from build123d import *

# Parameters (mm, degrees)
SKETCH1_W           = 736.6
SKETCH1_H           = 184.15
BOSS_EXTRUDE1_DEPTH = 38.1
CUT_EXTRUDE2_DEPTH  = 761.225224851
CHAMFER1_SIZE       = 2.54
CHAMFER2_SIZE       = 2.54
SKETCH2_R           = 19.05
CUT_EXTRUDE1_DEPTH  = 3.175


with BuildPart() as part:
    # Sketch1 → Boss-Extrude1 (new body)
    with BuildSketch(Plane(origin=(0, 0, 0), x_dir=(1, 0, 0), z_dir=(0, 1, 0))):
        with Locations((368.3, 92.075)):
            Rectangle(SKETCH1_W, SKETCH1_H)
        with BuildLine():
            Line((409.5623, 110.83925), (457.1238, 110.83925))
            ThreePointArc((457.1238, 110.83925), (469.8238, 98.13925), (457.1238, 85.43925))
            Line((457.1238, 85.43925), (409.5623, 85.43925))
            ThreePointArc((409.5623, 85.43925), (396.8623, 98.13925), (409.5623, 110.83925))
        make_face(mode=Mode.SUBTRACT)
    extrude(amount=BOSS_EXTRUDE1_DEPTH)

    # Sketch4 → Cut-Extrude2 (cut, through all)
    with BuildSketch(Plane.XZ):
        with BuildLine():
            Line((0, -184.15), (0, -113.957302712))
            ThreePointArc((0, -113.957302712), (2.738891811, -149.223945145), (8.343201677, -184.15))
            Line((8.343201677, -184.15), (0, -184.15))
        make_face()
    extrude(amount=-CUT_EXTRUDE2_DEPTH, mode=Mode.SUBTRACT)

    # Chamfer1
    # the kernel refuses this chamfer: 2.54 mm, written as the material it takes off along each edge
    with BuildSketch(Plane(origin=(736.6, 38.1, 6.532074789), x_dir=(0.027495876610568244, -0.9996219169112971, 0), z_dir=(0, 0, -1))) as chamfer1_piece_1:
        Polygon((CHAMFER1_SIZE * 0.999621916911, CHAMFER1_SIZE * 0.0274958766106), (-CHAMFER1_SIZE * 0.0274958766106, CHAMFER1_SIZE * 0.999621916911), (0, 0), align=None)
    extrude(amount=197.214149579, mode=Mode.SUBTRACT)
    with BuildSketch(Plane(origin=(457.1238, 38.1, -98.13925), x_dir=(0, 0, -1), z_dir=(-1, 0, 0))) as chamfer1_piece_2:
        Polygon((12.7 + CHAMFER1_SIZE, 0), (12.7, CHAMFER1_SIZE), (12.7, 0), align=None)
    revolve(axis=Axis((457.1238, 38.1, -98.13925), (0, -1, 0)), revolution_arc=180, mode=Mode.SUBTRACT)
    with BuildSketch(Plane(origin=(743.132074789, 38.1, -184.15), x_dir=(0, 0.027495876610587267, 0.9996219169112966), z_dir=(-1, 0, 0))) as chamfer1_piece_3:
        Polygon((CHAMFER1_SIZE * 0.999621916911, -CHAMFER1_SIZE * 0.0274958766106), (-CHAMFER1_SIZE * 0.0274958766106, -CHAMFER1_SIZE * 0.999621916911), (0, 0), align=None)
    extrude(amount=741.320947902, mode=Mode.SUBTRACT)
    with BuildSketch(Plane(origin=(409.5623, 38.1, -110.83925), x_dir=(0, 0.027495876610587267, -0.9996219169112966), z_dir=(1, 0, 0)), Plane(origin=(457.1238, 38.1, -85.43925), x_dir=(0, 0.027495876610587267, 0.9996219169112966), z_dir=(-1, 0, 0))) as chamfer1_piece_4:
        Polygon((CHAMFER1_SIZE * 0.999621916911, -CHAMFER1_SIZE * 0.0274958766106), (-CHAMFER1_SIZE * 0.0274958766106, -CHAMFER1_SIZE * 0.999621916911), (0, 0), align=None)
    extrude(amount=47.5615, mode=Mode.SUBTRACT)
    with BuildSketch(Plane(origin=(409.5623, 38.1, -98.13925), x_dir=(0, 0, 1), z_dir=(1, 0, 0))) as chamfer1_piece_5:
        Polygon((12.7 + CHAMFER1_SIZE, 0), (12.7, CHAMFER1_SIZE), (12.7, 0), align=None)
    revolve(axis=Axis((409.5623, 38.1, -98.13925), (0, -1, 0)), revolution_arc=180, mode=Mode.SUBTRACT)
    with BuildSketch(Plane(origin=(0, 38.1, -120.489377502), x_dir=(-0.02749587661058648, -0.9996219169112968, 0), z_dir=(0, 0, 1))) as chamfer1_piece_6:
        Polygon((CHAMFER1_SIZE * 0.999621916911, CHAMFER1_SIZE * 0.0274958766106), (-CHAMFER1_SIZE * 0.0274958766106, CHAMFER1_SIZE * 0.999621916911), (0, 0), align=None)
    extrude(amount=127.021452291, mode=Mode.SUBTRACT)
    with BuildSketch(Plane(origin=(433.324, 38.1, -98.044), x_dir=(-0.9997657983904642, 0, -0.021641357828885384), z_dir=(-0.021641357828885384, 0, 0.9997657983904642))) as chamfer1_piece_7:
        Polygon((433.6161 - CHAMFER1_SIZE, 0), (433.6161, CHAMFER1_SIZE), (433.6161, 0), align=None)
    revolve(axis=Axis((433.324, 38.1, -98.044), (0, -1, 0)), revolution_arc=11.076796252, mode=Mode.SUBTRACT)
    with BuildSketch(Plane(origin=(-6.532074789, 38.1, 0), x_dir=(0, -0.9996219169112968, 0.027495876610586393), z_dir=(1, 0, 0))) as chamfer1_piece_8:
        Polygon((CHAMFER1_SIZE * 0.999621916911, CHAMFER1_SIZE * 0.0274958766106), (-CHAMFER1_SIZE * 0.0274958766106, CHAMFER1_SIZE * 0.999621916911), (0, 0), align=None)
    extrude(amount=749.664149579, mode=Mode.SUBTRACT)

    # Chamfer2
    # the kernel refuses this chamfer: 2.54 mm, written as the material it takes off along each edge
    with BuildSketch(Plane(origin=(457.1238, 0, -98.13925), x_dir=(0, 0, -1), z_dir=(-1, 0, 0))) as chamfer2_piece_1:
        Polygon((12.7 + CHAMFER2_SIZE, 0), (12.7, -CHAMFER2_SIZE), (12.7, 0), align=None)
    revolve(axis=Axis((457.1238, 0, -98.13925), (0, -1, 0)), revolution_arc=180, mode=Mode.SUBTRACT)
    with BuildSketch(Plane(origin=(409.5623, 0, -110.83925), x_dir=(0, -0.027495876610586324, -0.9996219169112968), z_dir=(1, 0, 0)), Plane(origin=(457.1238, 0, -85.43925), x_dir=(0, -0.027495876610586324, 0.9996219169112968), z_dir=(-1, 0, 0))) as chamfer2_piece_2:
        Polygon((CHAMFER2_SIZE * 0.999621916911, CHAMFER2_SIZE * 0.0274958766106), (-CHAMFER2_SIZE * 0.0274958766106, CHAMFER2_SIZE * 0.999621916911), (0, 0), align=None)
    extrude(amount=47.5615, mode=Mode.SUBTRACT)
    with BuildSketch(Plane(origin=(409.5623, 0, -98.13925), x_dir=(0, 0, 1), z_dir=(1, 0, 0))) as chamfer2_piece_3:
        Polygon((12.7 + CHAMFER2_SIZE, 0), (12.7, -CHAMFER2_SIZE), (12.7, 0), align=None)
    revolve(axis=Axis((409.5623, 0, -98.13925), (0, -1, 0)), revolution_arc=180, mode=Mode.SUBTRACT)
    with BuildSketch(Plane(origin=(0, 0, -120.489377502), x_dir=(0.9996219169112968, -0.02749587661058605, 0), z_dir=(0, 0, 1))) as chamfer2_piece_4:
        Polygon((CHAMFER2_SIZE * 0.999621916911, CHAMFER2_SIZE * 0.0274958766106), (-CHAMFER2_SIZE * 0.0274958766106, CHAMFER2_SIZE * 0.999621916911), (0, 0), align=None)
    extrude(amount=127.021452291, mode=Mode.SUBTRACT)
    with BuildSketch(Plane(origin=(433.324, 0, -98.044), x_dir=(-0.9997657983904642, 0, -0.021641357828885415), z_dir=(-0.021641357828885415, 0, 0.9997657983904642))) as chamfer2_piece_5:
        Polygon((433.6161 - CHAMFER2_SIZE, 0), (433.6161, -CHAMFER2_SIZE), (433.6161, 0), align=None)
    revolve(axis=Axis((433.324, 0, -98.044), (0, -1, 0)), revolution_arc=11.076796252, mode=Mode.SUBTRACT)
    with BuildSketch(Plane(origin=(743.132074789, 0, -184.15), x_dir=(0, -0.027495876610586403, 0.9996219169112968), z_dir=(-1, 0, 0))) as chamfer2_piece_6:
        Polygon((CHAMFER2_SIZE * 0.999621916911, CHAMFER2_SIZE * 0.0274958766106), (-CHAMFER2_SIZE * 0.0274958766106, CHAMFER2_SIZE * 0.999621916911), (0, 0), align=None)
    extrude(amount=741.320947902, mode=Mode.SUBTRACT)
    with BuildSketch(Plane(origin=(736.6, 0, 6.532074789), x_dir=(-0.9996219169112966, -0.027495876610587444, 0), z_dir=(0, 0, -1))) as chamfer2_piece_7:
        Polygon((CHAMFER2_SIZE * 0.999621916911, CHAMFER2_SIZE * 0.0274958766106), (-CHAMFER2_SIZE * 0.0274958766106, CHAMFER2_SIZE * 0.999621916911), (0, 0), align=None)
    extrude(amount=197.214149579, mode=Mode.SUBTRACT)
    with BuildSketch(Plane(origin=(-6.532074789, 0, 0), x_dir=(0, 0.9996219169112968, 0.027495876610586407), z_dir=(1, 0, 0))) as chamfer2_piece_8:
        Polygon((CHAMFER2_SIZE * 0.999621916911, -CHAMFER2_SIZE * 0.0274958766106), (-CHAMFER2_SIZE * 0.0274958766106, -CHAMFER2_SIZE * 0.999621916911), (0, 0), align=None)
    extrude(amount=749.664149579, mode=Mode.SUBTRACT)

    # Sketch2 → Cut-Extrude1 (cut)
    with BuildSketch(Plane(origin=(0, 38.1, 0), x_dir=(1, 0, 0), z_dir=(0, 1, 0))):
        with Locations((433.34305, 98.13925)):
            Circle(SKETCH2_R)
    extrude(amount=-CUT_EXTRUDE1_DEPTH, mode=Mode.SUBTRACT)


solid = part.part
Source: CAD feature listing. Evaluate the final solid. Frame: model axes, mm. A direction names the side the tool comes from. Round coordinates to 2 decimals unless told otherwise and drop trailing zeros. One line per item, written item: value. Start each with the question number.
Item 1: Ray query, L1, parallel to Z at x = 409, y = 31; L2, parallel to Z at x = 467, y = 31.5; L3, parallel to X at y = 13.5, z = -123. Return the intervals inside material, ascending. Write a range as from..to.
Item 2: Set-up query: faces 1 (the flat face through (0, 19, -56)), 2 (the conical face through (469.94, 35.68, -98.42)), 3 (the cylindrical face through (469.82, 18.82, -98.42)), 4 (the flat face through (367, 19, -184.15)), 5 (the conical face through (469.94, 2.42, -98.42)). Return all of +Z, -Z, +X, -X, +Y, -Y with unobstructed straight access to the full face (end or side cutting, diameter ignored); none if empty.
Item 3: Mould query, pull axis Z, two halves, no side actions, for faces 6 (the cylindrical face through (396.865, 18.819, -97.86)), 7 (the cylindrical face through (2.68, 18.82, -148.73)), 8 (the flat face through (363, 19, 0)), 9 (the conical face through (396.742, 2.417, -97.857)). Classes: pulls with the +Z half, pulls with the -Z half, needs draft (parallel to the pull), parting line crosses it, or undercut.
Item 4: Pin query (flat end, axial travel): pin 1 (1.9 mm diameter, centred on x = 436.5, z = -115, fed in from +Y) (3 decimals). Return the tip coordinate at first contact, or that it passes through.
Result set:
1. L1: z = -184.15..-110.83, -85.45..0
1. L2: z = -184.15..-106.12, -90.15..0
1. L3: x = 0.43..736.6
2. face 1: +Z, -Z, -X, +Y, -Y
2. face 2: +Y
2. face 3: +Y, -Y
2. face 4: -Z, +X, -X, +Y, -Y
2. face 5: -Y
3. face 6: undercut
3. face 7: pulls with the -Z half
3. face 8: pulls with the +Z half
3. face 9: undercut
4. pin 1: stops at y = 34.925
